Autodesk Inventor part; units mm, degrees
ref_plane "YZ Plane" through (0, 0, 0) normal (1, 0, 0) x (0, 1, 0)
ref_plane "XZ Plane" through (0, 0, 0) normal (0, 1, 0) x (-1, 0, 0)
ref_plane "XY Plane" through (0, 0, 0) normal (0, 0, 1) x (1, 0, 0)
sketch "Sketch1" plane through (0, 0, 0) normal (0, 0, 1) x (1, 0, 0)
  line L0 (0, 63.5) -> (50.8, 63.5)
  line L1 (50.8, 63.5) -> (50.8, 6.35)
  line L2 (50.8, 6.35) -> (0, 6.35)
  line L3 (0, 6.35) -> (0, 63.5)
  dimension "d25" = 50.8
  dimension "d26" = 57.15
extrude "Extrusion4" add sketch "Sketch1" along normal blind 6.35
sketch "Sketch3" plane through (0, 0, 6.35) normal (0, 0, 1) x (1, 0, 0)
  line L0 (0, 63.5) -> (50.8, 63.5)
  line L1 (0, 6.35) -> (0, 63.5)
  circle A0 centre (25.4, 34.45) radius 10.625
  dimension "d29" = 21.25
  dimension "d30" = 25.4
  dimension "d31" = 29.05
extrude "Extrusion5" cut sketch "Sketch3" against normal through all
sketch "Sketch4" plane through (0, 0, 6.35) normal (0, 0, 1) x (1, 0, 0)
  line L0 (0, 63.5) -> (50.8, 63.5)
  line L1 (0, 6.35) -> (0, 63.5)
  circle A0 centre (3.49, 34.45) radius 1.6002
  circle A1 centre (47.32, 34.45) radius 1.6002
  circle A2 centre (25.4, 12.54) radius 1.6002
  dimension "d37" = 3.2004
  dimension "d38" = 3.49
  dimension "d39" = 29.05
  dimension "d40" = 3.2004
  dimension "d41" = 47.32
  dimension "d42" = 29.05
  dimension "d43" = 3.2004
  dimension "d44" = 25.4
  dimension "d45" = 50.96
extrude "Extrusion6" cut sketch "Sketch4" against normal through all
sketch "Sketch5" plane through (0, 0, 6.35) normal (0, 0, 1) x (1, 0, 0)
  line L0 (0, 63.5) -> (50.8, 63.5)
  line L1 (0, 6.35) -> (0, 63.5)
  arc A0 (12.9, 50.8) -> (17.9, 50.8) centre (15.4, 50.8) ccw
  line L2 (50.8, 6.35) -> (0, 6.35)
  line L3 (12.9, 50.8) -> (12.9, 57.8)
  line L4 (17.9, 50.8) -> (17.9, 57.8)
  arc A1 (17.9, 57.8) -> (12.9, 57.8) centre (15.4, 57.8) ccw
  dimension "d49" = 5
  dimension "d51" = 12.7
  dimension "d53" = 15.4
  dimension "d62" = 7
  dimension "d63" = 7
  dimension "d64" = 5
extrude "Extrusion7" cut sketch "Sketch5" against normal through all
pattern_linear "Rectangular Pattern1" count 2 spacing 20 along (1, 0, 0) of "Extrusion7"
fillet "Fillet1" radius 3.175 4 edges at (0, 63.5, 3.175) (50.8, 63.5, 3.175) (50.8, 6.35, 3.175) (0, 6.35, 3.175)
equation "\"d40\" = d37"
equation "\"d42\" = d39"
equation "\"d43\" = d37"
equation "\"d49\" = d48"
equation "\"d63\" = d62"
properties part number "SM-S06" material "Polycarbonate, Smoke"
Model file for the job. Use its own axes, mm. A direction names the side the tool comes from. Give positions to 0.01 mm unless a question says otherwise; leave off trailing zeros. Loops run counter-clockwise (first coordinate to the right, second up) from the corner with the lowest first, then second, coordinate; pieces in that order, holes last. Notation, with made-up numbers: (81, 57.25) - (118, 57.25) arc R16 cw to (118, 84.25) - close; hole circle Ø10 at (52, 58.5). An arc over 180 degrees is marked (long way). Use one line per item in the form item = value.
(1) Cut at B-B (y = 54.5). Give the cut face in (x, z).
Determined:
outline = (0, 0) - (12.9, 0) - (12.9, 6.35) - (0, 6.35) - close; (17.9, 0) - (32.9, 0) - (32.9, 6.35) - (17.9, 6.35) - close; (37.9, 0) - (50.8, 0) - (50.8, 6.35) - (37.9, 6.35) - close
(2) 3-axis set-ups, long thin cutter, end or side, ignore diameter. For faces 5 (the face through (0.91, 7.3, 3.22)), 6 (the face through (15.5, 60.3, 3.2)): which of +Z, -Z, +X, -X, +Y, -Y reach the whole face in a straight line?
Determined:
face_5 = +Z, -Z, -X, -Y
face_6 = +Z, -Z
(3) Cut at A-A (x = 25.4). Give the cut face in (y, z) (3 decimals).
Determined:
outline = (6.35, 0) - (10.94, 0) - (10.94, 6.35) - (6.35, 6.35) - close; (14.14, 0) - (23.825, 0) - (23.825, 6.35) - (14.14, 6.35) - close; (45.075, 0) - (63.5, 0) - (63.5, 6.35) - (45.075, 6.35) - close
(4) Cut at D-D (y = 34.45). Give the cut face in (x, z) (3 decimals).
Determined:
outline = (0, 0) - (1.89, 0) - (1.89, 6.35) - (0, 6.35) - close; (5.09, 0) - (14.775, 0) - (14.775, 6.35) - (5.09, 6.35) - close; (36.025, 0) - (45.72, 0) - (45.72, 6.35) - (36.025, 6.35) - close; (48.92, 0) - (50.8, 0) - (50.8, 6.35) - (48.92, 6.35) - close
(5) Cut at C-C (z = 3.25). Give the cut face in (x, y) (3 decimals).
Determined:
outline = (0, 9.525) arc R3.175 ccw to (3.175, 6.35) - (47.625, 6.35) arc R3.175 ccw to (50.8, 9.525) - (50.8, 60.325) arc R3.175 ccw to (47.625, 63.5) - (3.175, 63.5) arc R3.175 ccw to (0, 60.325) - close; hole circle Ø3.2 at (3.49, 34.45); hole (12.9, 50.8) arc R2.5 ccw to (17.9, 50.8) - (17.9, 57.8) arc R2.5 ccw to (12.9, 57.8) - close; hole circle Ø21.25 at (25.4, 34.45); hole circle Ø3.2 at (25.4, 12.54); hole (32.9, 50.8) arc R2.5 ccw to (37.9, 50.8) - (37.9, 57.8) arc R2.5 ccw to (32.9, 57.8) - close; hole circle Ø3.2 at (47.32, 34.45)
(6) Drill centre lines: L1, parallel to Y at x = 25.4, z = 5 (3 decimals); L2, parallel to Y at x = 47.32, z = 4.5; L3, parallel to X at y = 60, z = 4. Where is each one in solid material? Low to high.
Determined:
L1 = 6.35 to 10.94, 14.14 to 23.825, 45.075 to 63.5
L2 = 6.35 to 32.85, 36.05 to 63.5
L3 = 0 to 14.21, 16.59 to 34.21, 36.59 to 50.8
(7) Drop a flat-ended pin along its axis: P1, Ø1.9, axis at x = 25.4, y = 12.54, coming from the -Z side. Give the stop position or say it passes through.
Determined:
P1 = through
(8) Pull direction Y, two halves, no side cores. Call faces 1 (the face through (15.3, 48.3, 3.2)), 2 (the face through (3.282, 36.037, 3.219)), 3 (the face through (26, 6.35, 3)), 4 (the face through (36.3, 35.3, 0)): pulls with the +Y half, pulls with the -Y half, needs draft (parallel to the pull), parting line crosses it, or undercut.
Determined:
face_1 = undercut
face_2 = undercut
face_3 = pulls with the -Y half
face_4 = needs draft
